Part model, mm, in its own coordinate system. Face numbers are marked on the shaded views. A direction names the side the tool comes from. Coordinates: 2 decimals unless noted, no trailing zeros. Loops run counter-clockwise (first coordinate to the right, second up) from the corner with the lowest first, then second, coordinate; pieces in that order, holes last. Notation, with made-up numbers: M -35,75.5 L 9,75.5 A12 cw 9,87.5 Z; hole C -1,48.5 d4. An arc over 180 degrees is marked long. Use a Markdown table: item, result. Add a question column.
1) Band-saw the part on A-A (y = 0). List the corners of the cut face in (x, z) (3 decimals), plus the area to 3 significant figures.
2) Band-saw the part on C-C (x = -43). List the corners of the cut face in (y, z).
3) Pull direction Y, two halves, no side cores. Call the marked faces 3, 4 and 5: released by +Y, released by -Y, zero draft, split by the parting line, or undercut.
4) Band-saw the part on D-D (x = -31.75). List the corners of the cut face in (y, z), plus the area to 3 significant figures.
5) Wall check: probe 1 along Y at (x, z) = (-43.15, 38.45); probe 2 along Y at (x, z) = (-39.25, 43); probe 3 along Z at (x, y) = (-41, 6.25). Give the ranges that are in metal, low to high. Write a range as from..to.
6) Pin check, flat tips, straight feed: pin 1 Ø4 at (y, z) = (-7.5, 38.45) entering from +X (3 decimals); pin 2 Ø2 at (x, y) = (-27.5, 12) entering from +Z; pin 3 Ø1.7 at (x, y) = (-37, -7.5) entering from +Z. Stop position of each tip, or through.
7) Tool access for the marked faces 1 and 2: list every direction of +Z, -Z, +X, -X, +Y, -Y with a clear straight run to the whole face (end or side of a thin tool).
8) Band-saw the part on B-B (z = 38.45). List the corners of the cut face in (x, y) (3 decimals).
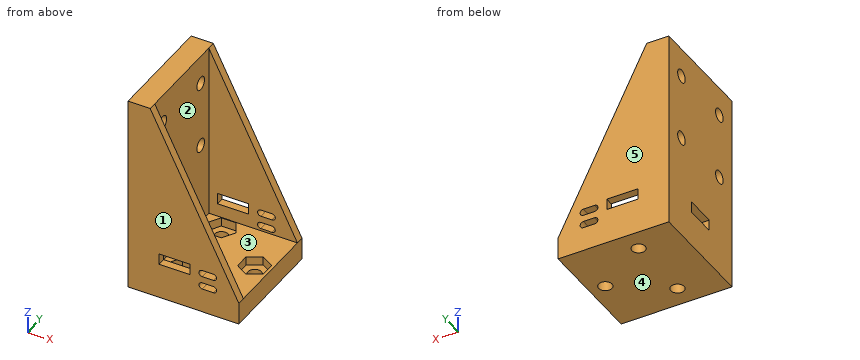
from build123d import *

# Parameters (mm, degrees)
SKETCH1_W           = 25
SKETCH1_H           = 25
SKETCH1_R           = 1.5
BOSS_EXTRUDE1_DEPTH = 5
SKETCH2_W           = 5
SKETCH2_H           = 25
BOSS_EXTRUDE2_DEPTH = 40
CUT_EXTRUDE1_DEPTH  = 2
BOSS_EXTRUDE3_DEPTH = 1.8
BOSS_EXTRUDE4_DEPTH = 1.8
SKETCH6_W           = 7
SKETCH6_H           = 2.5
CUT_EXTRUDE2_DEPTH  = 26
SKETCH7_W           = 2.5
SKETCH7_H           = 7
CUT_EXTRUDE3_DEPTH  = 6
CUT_EXTRUDE4_DEPTH  = 26
SKETCH9_R           = 1.5
CUT_EXTRUDE5_DEPTH  = 26


with BuildPart() as part:
    # Sketch1 → Boss-Extrude1 (new body)
    with BuildSketch(Plane.XY):
        with Locations((-32.675, 0)):
            Rectangle(SKETCH1_W, SKETCH1_H)
        with Locations((-35.625, 7.7)):
            Circle(SKETCH1_R, mode=Mode.SUBTRACT)
        with Locations((-35.625, -7.7)):
            Circle(SKETCH1_R, mode=Mode.SUBTRACT)
        with Locations((-23.725, 0)):
            Circle(SKETCH1_R, mode=Mode.SUBTRACT)
    extrude(amount=BOSS_EXTRUDE1_DEPTH)

    # Sketch2 → Boss-Extrude2 (add)
    with BuildSketch(Plane.XY.offset(5)):
        with Locations((-42.675, 0)):
            Rectangle(SKETCH2_W, SKETCH2_H)
    extrude(amount=BOSS_EXTRUDE2_DEPTH)

    # Sketch3 → Cut-Extrude1 (cut)
    with BuildSketch(Plane.XY.offset(5)):
        Polygon((-37.299315781, 4.8), (-33.950684219, 4.8), (-32.276368439, 7.7), (-33.950684219, 10.6), (-37.299315781, 10.6), (-38.973631561, 7.7), align=None)
        Polygon((-33.950684219, -4.8), (-37.299315781, -4.8), (-38.973631561, -7.7), (-37.299315781, -10.6), (-33.950684219, -10.6), (-32.276368439, -7.7), align=None)
        Polygon((-23.725, -3.348631561), (-20.825, -1.674315781), (-20.825, 1.674315781), (-23.725, 3.348631561), (-26.625, 1.674315781), (-26.625, -1.674315781), align=None)
    extrude(amount=-CUT_EXTRUDE1_DEPTH, mode=Mode.SUBTRACT)

    # Sketch4 → Boss-Extrude3 (add)
    with BuildSketch(Plane.XZ.offset(12.5)):
        Polygon((-40.175, 45), (-20.175, 5), (-40.175, 5), align=None)
    extrude(amount=-BOSS_EXTRUDE3_DEPTH)

    # Sketch5 → Boss-Extrude4 (add)
    with BuildSketch(Plane(origin=(0, 12.5, 0), x_dir=(1, 0, 0), z_dir=(0, 1, 0))):
        Polygon((-40.175, -45), (-20.175, -5), (-40.175, -5), align=None)
    extrude(amount=-BOSS_EXTRUDE4_DEPTH)

    # Sketch6 → Cut-Extrude2 (cut, through all)
    with BuildSketch(Plane(origin=(0, 12.5, 0), x_dir=(1, 0, 0), z_dir=(0, 1, 0))):
        with Locations((-34.675, -9.25)):
            Rectangle(SKETCH6_W, SKETCH6_H)
    extrude(amount=-CUT_EXTRUDE2_DEPTH, mode=Mode.SUBTRACT)

    # Sketch7 → Cut-Extrude3 (cut, through all)
    with BuildSketch(Plane(origin=(-40.175, 0, 0), x_dir=(0, 0, -1), z_dir=(1, 0, 0))):
        with Locations((-9.25, 0)):
            Rectangle(SKETCH7_W, SKETCH7_H)
    extrude(amount=-CUT_EXTRUDE3_DEPTH, mode=Mode.SUBTRACT)

    # Sketch8 → Cut-Extrude4 (cut, through all)
    with BuildSketch(Plane.XZ.offset(12.5)):
        with BuildLine():
            Line((-25.925, 10), (-28.425, 10))
            ThreePointArc((-28.425, 10), (-29.175, 9.25), (-28.425, 8.5))
            Line((-28.425, 8.5), (-25.925, 8.5))
            ThreePointArc((-25.925, 8.5), (-25.175, 9.25), (-25.925, 10))
        make_face()
        with BuildLine():
            Line((-28.425, 5.5), (-25.925, 5.5))
            ThreePointArc((-25.925, 5.5), (-25.175, 6.25), (-25.925, 7))
            Line((-25.925, 7), (-28.425, 7))
            ThreePointArc((-28.425, 7), (-29.175, 6.25), (-28.425, 5.5))
        make_face()
    extrude(amount=-CUT_EXTRUDE4_DEPTH, mode=Mode.SUBTRACT)

    # Sketch9 → Cut-Extrude5 (cut, through all)
    with BuildSketch(Plane.ZY.offset(45.175)):
        with Locations((23.45, 7.5)):
            Circle(SKETCH9_R)
        with Locations((23.45, -7.5)):
            Circle(SKETCH9_R)
        with Locations((38.45, 7.5)):
            Circle(SKETCH9_R)
        with Locations((38.45, -7.5)):
            Circle(SKETCH9_R)
    extrude(amount=-CUT_EXTRUDE5_DEPTH, mode=Mode.SUBTRACT)


solid = part.part
Entries:
| question | item | result |
|---|---|---|
| 1 | outline | M -45.175,0 L -25.225,0 L -25.225,3 L -26.625,3 L -26.625,5 L -40.175,5 L -40.175,8 L -45.175,8 Z; M -45.175,10.5 L -40.175,10.5 L -40.175,45 L -45.175,45 Z; M -22.225,0 L -20.175,0 L -20.175,5 L -20.825,5 L -20.825,3 L -22.225,3 Z |
| 1 | area | 292 mm2 |
| 2 | outline | M -12.5,0 L 12.5,0 L 12.5,45 L -12.5,45 Z; hole C -7.5,23.45 d3; hole C -7.5,38.45 d3; hole M -3.5,8 L 3.5,8 L 3.5,10.5 L -3.5,10.5 Z; hole C 7.5,23.45 d3; hole C 7.5,38.45 d3 |
| 3 | face 3 | undercut |
| 3 | face 4 | zero draft |
| 3 | face 5 | released by +Y |
| 4 | outline | M -12.5,0 L 12.5,0 L 12.5,8 L 10.7,8 L 10.7,5 L -10.7,5 L -10.7,8 L -12.5,8 Z; M -12.5,10.5 L -10.7,10.5 L -10.7,28.15 L -12.5,28.15 Z; M 10.7,10.5 L 12.5,10.5 L 12.5,28.15 L 10.7,28.15 Z |
| 4 | area | 199 mm2 |
| 5 | probe 1 | -12.5..-9, -6..6, 9..12.5 |
| 5 | probe 2 | -12.5..-10.7, 10.7..12.5 |
| 5 | probe 3 | 0..22.62, 24.28..37.62, 39.28..45 |
| 6 | pin 1 | x = -40.175 |
| 6 | pin 2 | z = 21.65 |
| 6 | pin 3 | z = 3 |
| 7 | face 1 | +Z, -Z, +X, -X, -Y |
| 7 | face 2 | +Z, +X |
| 8 | outline | M -45.175,-12.5 L -36.9,-12.5 L -36.9,-10.7 L -40.175,-10.7 L -40.175,-9 L -45.175,-9 Z; M -45.175,-6 L -40.175,-6 L -40.175,6 L -45.175,6 Z; M -45.175,9 L -40.175,9 L -40.175,10.7 L -36.9,10.7 L -36.9,12.5 L -45.175,12.5 Z |
